Geometry: final body of the model. Coordinates: model frame, mm. Give positions to 0.01 mm unless a question says otherwise; leave off trailing zeros. Order: outer loops, then holes, each group sorted by start corner. A loop starts at its lowest first (then second) coordinate and runs counter-clockwise, first axis right, second up. Notation, with made-up numbers: M 30,60 L 66,60 A24 cw 66,74 Z; hole C -38,-30.75 d11. An arc over 180 degrees is marked long. Write item = value, one per line. Start each with the question number.
from build123d import *

# Parameters (mm, degrees)
SKETCH_1_R      = 1.5
EXTRUDE_1_DEPTH = 3
FILLET_1_R      = 10
FILLET_2_R      = 2
FILLET_3_R      = 2


with BuildPart() as part:
    # 草图1 → 凸台-拉伸1 (new body)
    with BuildSketch(Plane(origin=(0, 0, 0), x_dir=(1, 0, 0), z_dir=(0, 1, 0))):
        Polygon((0, 110), (0, 129.5), (8, 129.5), (26.335454545, 8), (33.6, 8), (33.6, 0), (16.6, 0), align=None)
        with Locations(Location((21.1, 4, 0), (0, 0, 270))):
            Circle(SKETCH_1_R, mode=Mode.SUBTRACT)
        with Locations(Location((29.1, 4, 0), (0, 0, 270))):
            Circle(SKETCH_1_R, mode=Mode.SUBTRACT)
        with Locations(Location((4, 115.5, 0), (0, 0, 270))):
            Circle(SKETCH_1_R, mode=Mode.SUBTRACT)
        with Locations(Location((4, 123.5, 0), (0, 0, 270))):
            Circle(SKETCH_1_R, mode=Mode.SUBTRACT)
    extrude(amount=EXTRUDE_1_DEPTH)

    # 圆角1
    # the kernel refuses this fillet: 10 mm, written as the material it adds along each edge
    with BuildSketch(Plane(origin=(26.335454545, 0, -8), x_dir=(-0.1492195266498612, 0, -0.9888040922581132), z_dir=(0, 1, 0))) as fillet_1_piece_1:
        with BuildLine():
            CenterArc((8.51107561, -10), FILLET_1_R, 90, 73.639575316)
            Line((-1.084012034, -7.183212274), (-1.275913787, -7.126876519))
            ThreePointArc((-1.275913787, -7.126876519), (-0.739766835, -3.561762232), (-0.197760818, 0.029843905))
            Line((-0.197760818, 0.029843905), (0, 0.2))
            Line((0, 0.2), (8.51107561, 0.2))
            Line((8.51107561, 0.2), (8.51107561, 0))
        make_face()
    extrude(amount=3)

    # 圆角2
    fillet_2_edges = [part.edges().sort_by_distance(p)[0] for p in [
        (0, 1.5, -129.5),
        (8, 1.5, -129.5),
        (33.6, 1.5, 0),
        (16.6, 1.5, 0),
    ]]
    fillet(fillet_2_edges, radius=FILLET_2_R)

    # 圆角3
    fillet_3_edges = [part.edges().sort_by_distance(p)[0] for p in [
        (33.6, 1.5, -8),
    ]]
    fillet(fillet_3_edges, radius=FILLET_3_R)


solid = part.part
1) Ray query, L1, parallel to X at y = 0.65, z = -123; L2, parallel to X at y = 1.55, z = -4; L3, parallel to X at y = 2.2, z = -92. Return the intervals inside material, ascending.
2) Cut plane B-B (z = -123.5). Return loops of the section in (x, y), plus the area to 3 significant figures.
3) Cut plane C-C (x = 21.1). Return loops of the section in (y, z).
4) Cut plane D-D (z = -4). Return loops of the section in (x, y).
5) Cut plane A-A (y = 0.75). Return loops of the section in (x, z).
6) Draft query along X for faces 1 (the cylindrical face through (4, 1, -117)), 2 (the flat face through (16.543, 1.479, -72.887)), 3 (the flat face through (0, 1, -119)). Return one class per face: pulls with the +X half, pulls with the -X half, needs draft (parallel to the pull), parting line crosses it, or undercut.
Reply:
q1.L1 = 0 to 2.59, 5.41 to 8.98
q1.L2 = 16 to 19.6, 22.6 to 27.6, 30.6 to 33.6
q1.L3 = 2.72 to 13.66
q2.outline = M 0,0 L 2.5,0 L 2.5,3 L 0,3 Z; M 5.5,0 L 8.91,0 L 8.91,3 L 5.5,3 Z
q2.area = 17.7 mm²
q3.outline = M 0,-42.69 L 3,-42.69 L 3,-5.5 L 0,-5.5 Z; M 0,-2.5 L 3,-2.5 L 3,0 L 0,0 Z
q4.outline = M 16,0 L 19.6,0 L 19.6,3 L 16,3 Z; M 22.6,0 L 27.6,0 L 27.6,3 L 22.6,3 Z; M 30.6,0 L 33.6,0 L 33.6,3 L 30.6,3 Z
q5.outline = M 0,-127.5 A2 ccw 2,-129.5 L 6.28,-129.5 A2 ccw 8.26,-127.8 L 25.07,-16.42 A10 cw 32.16,-8.31 A2 ccw 33.6,-6.39 L 33.6,-2 A2 ccw 31.6,0 L 18.32,0 A2 ccw 16.34,-1.7 L 0,-110 Z; hole C 4,-123.5 d3; hole C 4,-115.5 d3; hole C 21.1,-4 d3; hole C 29.1,-4 d3
q6.face_1 = undercut
q6.face_2 = pulls with the +X half
q6.face_3 = pulls with the -X half
